Geometry: final body of the model. Coordinates: model frame, mm. Give positions to 0.01 mm unless a question says otherwise; leave off trailing zeros. Order: outer loops, then holes, each group sorted by start corner. A loop starts at its lowest first (then second) coordinate and runs counter-clockwise, first axis right, second up. Notation, with made-up numbers: (56.5, 79.25) - (104.5, 79.25) arc R19 cw to (104.5, 98.25) - close; hole circle Ø1 at (69, 87). An arc over 180 degrees is marked (long way). Use one line per item in the form item = value.
Autodesk Inventor part; units mm, degrees
ref_plane "YZ Plane" through (0, 0, 0) normal (1, 0, 0) x (0, 1, 0)
ref_plane "XZ Plane" through (0, 0, 0) normal (0, 1, 0) x (-1, 0, 0)
ref_plane "XY Plane" through (0, 0, 0) normal (0, 0, 1) x (1, 0, 0)
sketch "スケッチ1" plane through (0, 0, 0) normal (0, 0, 1) x (1, 0, 0)
  circle A0 centre (0, 0) radius 21.2
  circle A1 centre (0, 0) radius 7.5
  circle A2 centre (0, 0) radius 30
  circle A3 centre (20.819222, -21.6) radius 22.5
  circle A4 centre (20.819222, -21.6) radius 14
  circle A5 centre (20.819222, -21.6) radius 62
  circle A6 centre (0, -80) radius 48
  circle A7 centre (0, -80) radius 50
  circle A8 centre (20.819222, -21.6) radius 4
  circle A9 centre (0, -80) radius 4
  dimension "d2" = 60
  dimension "d4" = 124
  dimension "d0" = 42.4
  dimension "d1" = 15
  dimension "d3" = 28
  dimension "d5" = 100
  dimension "d23" = 8
  dimension "d41" = 8
sketch "スケッチ2" plane through (0, 0, 0) normal (0, 0, 1) x (1, 0, 0)
  line L0 (0, 0) -> (24.501973, 0) construction
  line L1 (0, 0) -> (12.5, 0) construction
  line L2 (0, 0) -> (10.253048, 10.253048)
  line L3 (0, 0) -> (14.5, 0) construction
  line L4 (10.253048, 10.253048) -> (-10.253048, -10.253048)
  circle A0 centre (10.253048, 10.253048) radius 2
  circle A1 centre (-10.253048, -10.253048) radius 2
  circle A2 centre (0, 0) radius 7.5
  line L5 (0, 0) -> (28.190779, 10.260604)
  line L6 (0, 0) -> (30, 0) construction
  line L7 (0, 0) -> (-28.190779, 10.260604)
  line L8 (0, 0) -> (30, 0) construction
  circle A3 centre (-28.190779, 10.260604) radius 2.5
  line L9 (0, 0) -> (0, 30)
  circle A4 centre (0, 30) radius 2.5
  circle A5 centre (28.190779, 10.260604) radius 2.5
  dimension "d9" = 14.5
  dimension "d10" = 45
  dimension "d11" = 29
  dimension "d12" = 4
  dimension "d13" = 4
  dimension "d14" = 15
  dimension "d15" = 30
  dimension "d16" = 20
  dimension "d17" = 30
  dimension "d18" = 160
  dimension "d19" = 5
  dimension "d20" = 30
  dimension "d21" = 5
  dimension "d22" = 5
sketch "スケッチ3" plane through (0, 0, 0) normal (0, 0, 1) x (1, 0, 0)
  line L0 (60, -99.343647) -> (-60, -99.343647)
  line L1 (-60, -99.343647) -> (-60, 99.343647)
  line L2 (-60, 99.343647) -> (60, 99.343647)
  line L3 (60, 99.343647) -> (60, -99.343647)
  line L4 (60, -99.343647) -> (-60, 99.343647) construction
  line L5 (-60, -99.343647) -> (60, 99.343647) construction
  point P0 (0, 0)
  dimension "d25" = 120
extrude "押し出し1" add sketch "スケッチ3" against normal blind 3
sketch "スケッチ4" plane through (0, 0, 0) normal (0, 0, 1) x (1, 0, 0)
  line L0 (0, 45.071117) -> (68.359536, 45.071117)
  line L1 (68.359536, 45.071117) -> (-74.382402, 45.071117)
  line L2 (-74.382402, 45.071117) -> (108.165644, 45.071117)
  line L3 (108.165644, 45.071117) -> (108.165644, 129.415375)
  line L4 (108.165644, 129.415375) -> (-74.382402, 129.415375)
  line L5 (-74.382402, 129.415375) -> (-74.382402, 45.071117)
  point P0 (0, 0)
extrude "押し出し4" cut sketch "スケッチ4" against normal blind 10
fillet "フィレット1" radius 4 4 edges at (-60, 45.0711, -1.5) (60, 45.0711, -1.5) (-60, -99.3436, -1.5) (60, -99.3436, -1.5)
extrude "押し出し7" cut sketch "スケッチ1" against normal blind 10 contours A8 A2 | A2 A8 | A9 A5 | A5 A9
extrude "押し出し9" cut sketch "スケッチ2" against normal blind 4 contours L9 A2 L2 | L5 A2 L4 | L2 A2 L5 | L4 A2 L7 | L7 A2 L9 | A0 | A1
equation "\"d46\" = d12"
properties part number "板"
(1) Cut plane B-B on y = -21.6. Output: boundary loops of the cut face in (x, z).
Computed values:
outline = (-60, -3) - (16.82, -3) - (16.82, 0) - (-60, 0) - close; (24.82, -3) - (60, -3) - (60, 0) - (24.82, 0) - close
(2) Cut plane C-C on y = 0. Output: boundary loops of the cut face in (x, z), plus the area to 3 significant figures.
Computed values:
outline = (-60, -3) - (-7.5, -3) - (-7.5, 0) - (-60, 0) - close; (7.5, -3) - (60, -3) - (60, 0) - (7.5, 0) - close
area = 315 mm²
(3) Pull-direction query (Y, two-part tool) for faces 1 (the face through (1, -99.344, -1)), 2 (the face through (20.299, -17.634, -1.479)), 3 (the face through (-1, -26, -3)); classes: released by +Y, released by -Y, zero draft, split by the parting line, or undercut.
Computed values:
face_1 = released by -Y
face_2 = undercut
face_3 = zero draft
(4) Cut plane D-D on z = -1.25. Output: boundary loops of the cut face in (x, y), plus the area to 3 significant figures.
Computed values:
outline = (-60, -95.34) arc R4 ccw to (-56, -99.34) - (56, -99.34) arc R4 ccw to (60, -95.34) - (60, 41.07) arc R4 ccw to (56, 45.07) - (-56, 45.07) arc R4 ccw to (-60, 41.07) - close; hole circle Ø4 at (-10.25, -10.25); hole circle Ø15 at (0, 0); hole circle Ø8 at (0, -80); hole circle Ø4 at (10.25, 10.25); hole circle Ø8 at (20.82, -21.6)
area = 17,000 mm²
(5) Cut plane A-A on x = 0. Output: boundary loops of the cut face in (y, z).
Computed values:
outline = (-99.34, -3) - (-84, -3) - (-84, 0) - (-99.34, 0) - close; (-76, -3) - (-7.5, -3) - (-7.5, 0) - (-76, 0) - close; (7.5, -3) - (45.07, -3) - (45.07, 0) - (7.5, 0) - close
(6) Contact query for flat-ended pins moving along their axis: pin 1 Ø1.5 at (x, y) = (24.5, -19.5) entering from +Z; pin 2 Ø2.5 at (x, y) = (-10.25, -10.25) entering from +Z. Output: stop coordinate, or through.
Computed values:
pin_1 = 0
pin_2 = through
(7) Ray query, line 1 along Y through (x, z) = (0, -1.15); line 2 along X through (y, z) = (-80, -1.95); line 3 along X through (y, z) = (-21.6, -0.6). Return the intervals inside material, ascending.
Computed values:
line_1 = -99.34 to -84, -76 to -7.5, 7.5 to 45.07
line_2 = -60 to -4, 4 to 60
line_3 = -60 to 16.82, 24.82 to 60
